Autodesk Inventor part; units mm, degrees
ref_plane "YZ Plane" through (0, 0, 0) normal (1, 0, 0) x (0, 1, 0)
ref_plane "XZ Plane" through (0, 0, 0) normal (0, 1, 0) x (-1, 0, 0)
ref_plane "XY Plane" through (0, 0, 0) normal (0, 0, 1) x (1, 0, 0)
sketch "Sketch1" plane through (0, 0, 0) normal (0, 0, 1) x (1, 0, 0)
  line L0 (0, 4.2) -> (0, -4.2)
  line L1 (-4.2, 0) -> (4.2, 0)
  circle A0 centre (0, 0) radius 3
  dimension "d0" = 6
extrude "Extrusion1" add sketch "Sketch1" along normal blind 20
chamfer "Chamfer1" distance 1 angle 30 1 edges at (-3, 0, 0) measured on face at (-0.5351, 1.0949, 0)
fillet "Fillet1" radius 0.5 1 edges at (-3, 0, 20)
sketch "Sketch2" plane through (0, 0, 20) normal (0, 0, 1) x (1, 0, 0)
  circle A0 centre (0, 0) radius 2.5
hole "Hole1" at (0, 0, 20) direction (0, 0, -1) diameter 3.242 depth 8 tip angle 118
chamfer "Chamfer2" distance 0.25 angle 45 1 edges at (0, 1.621, 20)
properties part number "PIN, DOWEL, PULL, 6MMODX20MM" material "Steel, 4140, Carb & Case Harden 58-60 Rc, 0.06 Dp Case"
Verification items for the finished model (mm, model axes). Coordinates: 2 decimals unless noted, no trailing zeros. Order: outer loops, then holes, each group sorted by start corner. A loop starts at its lowest first (then second) coordinate and runs counter-clockwise, first axis right, second up. Notation, with made-up numbers: (16, 13) - (45, 13) arc R28 ccw to (45, 37) - close; hole circle Ø6 at (54, 55.5). An arc over 180 degrees is marked (long way). Return JSON: item names as keys, results as strings.
(1) Go/stop test with flat-tipped pins: pin 1 (3 mm diameter, centred on x = 2, y = 1, fed in from -Z); pin 2 (3 mm diameter, centred on x = -2, z = 9, fed in from +Y); pin 3 (1.5 mm diameter, centred on y = 1, z = 17, fed in from +X). Record where each tip stops, or that it passes through.
Filled sheet:
{"pin 1": "stops at z = 0", "pin 2": "stops at y = 2.96", "pin 3": "stops at x = 2.99"}
(2) Section check B-B, the plane z = 3.5. Record the cut outline in (x, y), and give its area (3 significant figures).
Filled sheet:
{"outline": "circle Ø6 at (0, 0)", "area": "28.3 mm^2"}
(3) Mould release check, pull along X, two halves, no side actions. Record for faces 1 (the cylindrical face through (-3, 0, 10)), 2 (the flat face through (1, -2, 20)), 3 (the cylindrical face through (1.438, -0.748, 15.821)): pulls with the +X half, pulls with the -X half, needs draft (parallel to the pull), parting line crosses it, or undercut.
Filled sheet:
{"face 1": "parting line crosses it", "face 2": "needs draft", "face 3": "undercut"}
(4) Thickness scan on line 1 along Y through (x, z) = (0, 14); line 2 along X through (y, z) = (0.2, 11.75). Record the ranges inside material, lowest first.
Filled sheet:
{"line 1": "y = -3 to -1.62, 1.62 to 3", "line 2": "x = -2.99 to -1.19, 1.19 to 2.99"}
(5) Section check A-A, the plane z = 13.75. Record the cut outline in (x, y).
Filled sheet:
{"outline": "circle Ø6 at (0, 0); hole circle Ø3.24 at (0, 0)"}
